from build123d import *

# Parameters (mm, degrees)
F1_DEPTH = 63.5
F0_W     = 25.4
F0_H     = 19.05
F2_DEPTH = 25.4
F3_DEPTH = 7.9375
F5_R     = 5.08


with BuildPart() as f1:
    # F0 (on Front) → F1 (new body, symmetric)
    with BuildSketch(Plane.XZ):
        Polygon((41.275, -9.525), (41.275, 9.525), (22.225, 9.525), (-41.275, 9.525), (-41.275, -9.525), align=None)
    extrude(amount=F1_DEPTH, both=True)

    # F0 (on Front) → F2 (join, symmetric)
    with BuildSketch(Plane.XZ):
        with BuildLine():
            Line((22.225, 9.525), (41.275, 9.525))
            Line((41.275, 9.525), (41.275, 27.0002))
            ThreePointArc((41.275, 27.0002), (45.9246798487, 38.2255201513), (57.15, 42.8752))
            Line((57.15, 42.8752), (60.325, 42.8752))
            Line((60.325, 42.8752), (60.325, 61.9252))
            Line((60.325, 61.9252), (57.15, 61.9252))
            add(Edge.make_bspline(
                [(55.1065701704, 61.8653691453), (55.7928245706, 61.8885825156), (56.4740931421, 61.9085013809), (57.15, 61.9252)],
                knots=[109.6237509197, 109.6237509197, 109.6237509197, 109.6237509197, 111.5045361635, 111.5045361635, 111.5045361635, 111.5045361635], degree=3))
            ThreePointArc((55.1065701704, 61.8653691453), (31.7421034735, 50.9625542062), (22.225, 27.0002))
            Line((22.225, 27.0002), (22.225, 9.525))
        make_face()
        with Locations((73.025, 52.4002)):
            Rectangle(F0_W, F0_H)
    extrude(amount=F2_DEPTH, both=True)

    # F0 (on Front) → F3 (join, symmetric)
    with BuildSketch(Plane.XZ):
        with BuildLine():
            Line((-41.275, 9.525), (22.225, 9.525))
            Line((22.225, 9.525), (22.225, 27.0002))
            ThreePointArc((22.225, 27.0002), (31.7421034735, 50.9625542062), (55.1065701704, 61.8653691453))
            add(Edge.make_bspline(
                [(-41.275, 9.525), (-41.8299371409, 47.9669883241), (15.1074359349, 60.5123509154), (55.1065701704, 61.8653691453)],
                knots=[0, 0, 0, 0, 109.6237509197, 109.6237509197, 109.6237509197, 109.6237509197], degree=3))
        make_face()
    extrude(amount=F3_DEPTH, both=True)

    # F0 (on Front) → F4 (revolve)
    with BuildSketch(Plane.XZ):
        Polygon((85.725, 61.9252), (85.725, 42.8752), (85.725, 38.1), (111.125, 38.1), (111.125, 66.675), (85.725, 66.675), align=None)
    revolve(axis=Axis((85.725, 0, 52.3875), (0, 0, 1)))

    # F5
    f5_edges = [f1.edges().sort_by_distance(p)[0] for p in [
        (41.275, -63.5, 0),
        (-41.275, -63.5, 0),
        (-41.275, 63.5, 0),
        (41.275, 63.5, 0),
    ]]
    fillet(f5_edges, radius=F5_R)


solid = f1.part
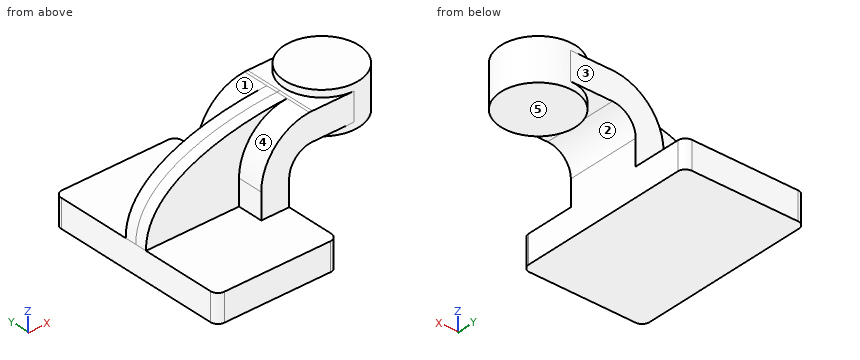
CAD build for the part. Positions are in the model's coordinates, mm. Face numbers are marked on the shaded views. A direction names the side the tool comes from. Round coordinates to 2 decimals unless told otherwise and drop trailing zeros. Loops run counter-clockwise (first coordinate to the right, second up) from the corner with the lowest first, then second, coordinate; pieces in that order, holes last. Notation, with made-up numbers: M 21,71 L 27,71 A15 ccw 27,81 Z; hole C 61,43.5 d1. An arc over 180 degrees is marked long. One line per question, with ' | ' between items. Start each with the question number.
Item 1: Pin check, flat tips, straight feed: pin 1 Ø6 at (x, y) = (51.5, 1.5) entering from +Z; pin 2 Ø3 at (x, z) = (-8, 42.5) entering from -Y; pin 3 Ø21 at (y, z) = (-13.5, -1.5) entering from -X (3 decimals). Stop position of each tip, or through.
Item 2: Cut at B-B, the plane x = 80.5. Write the cut outline in (y, z) (3 decimals).
Item 3: Wall check: line 1 (X direction, y = -54, z = 8.5) (3 decimals); line 2 (Y direction, x = -31.5, z = 15); line 3 (Z direction, x = 25.5, y = 38) (3 decimals). Give the ranges that are in metal, low to high.
Item 4: Which spindle directions (+Z, -Z, +X, -X, +Y, -Y) get a long thin tool onto all of the face, cutting with end or side? Do the marked faces 1, 2, 3, 4 and 5. Say none if no direction does.
Item 5: Cut at A-A, the plane z = 5. Write the cut outline in (x, y) (3 decimals).
Item 6: Cut at C-C, the plane y = -50. Write the cut outline in (x, z) (3 decimals), plus the area to 3 significant figures.
Responses:
1) pin 1: stops at z = 61.84 | pin 2: stops at y = -7.94 | pin 3: stops at x = -41.275
2) outline: M -25.4,42.875 L -24.857,42.875 L -24.857,38.1 L 24.857,38.1 L 24.857,42.875 L 25.4,42.875 L 25.4,61.925 L 24.857,61.925 L 24.857,66.675 L -24.857,66.675 L -24.857,61.925 L -25.4,61.925 Z
3) line 1: x = -41.275 to 41.275 | line 2: y = -7.94 to 7.94 | line 3: z = -9.525 to 9.525
4) face 1: +Z, -X, +Y | face 2: -Z, +Y, -Y | face 3: +Z, +X, -X, +Y | face 4: +Z, -X, -Y | face 5: -Z, +X, +Y, -Y
5) outline: M -41.275,-58.42 A5.08 ccw -36.195,-63.5 L 36.195,-63.5 A5.08 ccw 41.275,-58.42 L 41.275,58.42 A5.08 ccw 36.195,63.5 L -36.195,63.5 A5.08 ccw -41.275,58.42 Z
6) outline: M -41.275,-9.525 L 41.275,-9.525 L 41.275,9.525 L -41.275,9.525 Z | area: 1,570 mm²
